from build123d import *

# Parameters (mm, degrees)
F0_R     = 2
F0_R_2   = 2.5
F2_DEPTH = 25


# Not quite as in the source:
# - ends of sketch curves that miss each other by under 0.0002 mm in the source are joined


with BuildPart() as f2:
    # F0 (on Front) → F2 (new body)
    with BuildSketch(Plane.XZ):
        with BuildLine():
            ThreePointArc((5.2500001607, 6.6439288361), (0, 4.5), (-5.2500001607, 6.6439288361))
            Line((-5.2500001607, 6.6439288361), (-5.25, 10.5))
            Line((-5.25, 10.5), (-3.375, 10.5))
            Line((-3.375, 10.5), (-3.375, 12.5))
            Line((-3.375, 12.5), (-7.5, 12.5))
            ThreePointArc((-7.5, 12.5), (-11.0355339059, 11.0355339059), (-12.5, 7.5))
            Line((-12.5, 7.5), (-12.5, 3.375))
            Line((-12.5, 3.375), (-10.5, 3.375))
            Line((-10.5, 3.375), (-10.5, 5.25))
            Line((-10.5, 5.25), (-6.643929, 5.25))
            ThreePointArc((-6.643929, 5.25), (-4.5, 0), (-6.6439288361, -5.2500001607))
            Line((-6.6439288361, -5.2500001607), (-10.5, -5.25))
            Line((-10.5, -5.25), (-10.5, -3.375))
            Line((-10.5, -3.375), (-12.5, -3.375))
            Line((-12.5, -3.375), (-12.5, -7.5))
            ThreePointArc((-12.5, -7.5), (-11.0355339059, -11.0355339059), (-7.5, -12.5))
            Line((-7.5, -12.5), (-3.375, -12.5))
            Line((-3.375, -12.5), (-3.375, -10.5))
            Line((-3.375, -10.5), (-5.25, -10.5))
            Line((-5.25, -10.5), (-5.25, -6.643929))
            ThreePointArc((-5.25, -6.643929), (0, -4.5), (5.2500001607, -6.6439288361))
            Line((5.2500001607, -6.6439288361), (5.25, -10.5))
            Line((5.25, -10.5), (3.375, -10.5))
            Line((3.375, -10.5), (3.375, -12.5))
            Line((3.375, -12.5), (7.5, -12.5))
            ThreePointArc((7.5, -12.5), (11.0355339059, -11.0355339059), (12.5, -7.5))
            Line((12.5, -7.5), (12.5, -3.375))
            Line((12.5, -3.375), (10.5, -3.375))
            Line((10.5, -3.375), (10.5, -5.25))
            Line((10.5, -5.25), (6.643929, -5.25))
            ThreePointArc((6.643929, -5.25), (4.5, 0), (6.6439288361, 5.2500001607))
            Line((6.6439288361, 5.2500001607), (10.5, 5.25))
            Line((10.5, 5.25), (10.5, 3.375))
            Line((10.5, 3.375), (12.5, 3.375))
            Line((12.5, 3.375), (12.5, 7.5))
            ThreePointArc((12.5, 7.5), (11.0355339059, 11.0355339059), (7.5, 12.5))
            Line((7.5, 12.5), (3.375, 12.5))
            Line((3.375, 12.5), (3.375, 10.5))
            Line((3.375, 10.5), (5.25, 10.5))
            Line((5.25, 10.5), (5.2500001607, 6.6439288361))
        make_face()
        with Locations((-8.5, -8.5)):
            Circle(F0_R, mode=Mode.SUBTRACT)
        with Locations((8.5, -8.5)):
            Circle(F0_R, mode=Mode.SUBTRACT)
        with Locations((-8.5, 8.5)):
            Circle(F0_R, mode=Mode.SUBTRACT)
        Circle(F0_R_2, mode=Mode.SUBTRACT)
        with Locations((8.5, 8.5)):
            Circle(F0_R, mode=Mode.SUBTRACT)
    extrude(amount=F2_DEPTH)


solid = f2.part
Work out the finished part from the listing and answer in its coordinate system (mm). A direction names the side the tool comes from. Round coordinates to 2 decimals unless told otherwise and drop trailing zeros. Write each loop counter-clockwise with the first axis right and the second up, starting at its lowest first coordinate (ties: lowest second). Pieces come first, ordered by that corner, then holes.
1) A cutting plane is placed at A-A (x = 0). Give the vertices of the cut face in (y, z).
2) Given pin 1 Ø1 at (y, z) = (-14.5, 11.5) entering from +X; pin 2 Ø1.2 at (x, y) = (9, -8) entering from -Z; pin 3 Ø1.6 at (y, z) = (-8.5, -12) entering from -X, each flat-ended and moving along its own axis, determine where each tip first touches the part or whether it passes through.
3) A cutting plane is placed at D-D (z = 0). Give the vertices of the cut face in (x, y).
4) A cutting plane is placed at B-B (z = -8.5). Give the vertices of the cut face in (x, y).
5) The mould has two halves that part along X. Classify faces 5 (the cylindrical face through (11, -12.32, -11.07)), 6 (the flat face through (5.25, -12, -9)), 7 (the flat face through (-5, -12, -12.5)): pulls with the +X half, pulls with the -X half, needs draft (parallel to the pull), parting line crosses it, or undercut.
6) A tool of negligible diameter and unlimited length cuts with its end or side. For faces 1 (the flat face through (11, -12, 3.375)), 2 (the flat face through (-3.375, -12, -12)), 3 (the flat face through (-5.25, -12, 9)), 4 (the flat face through (3.375, -12, 12)), from which of +Z, -Z, +X, -X, +Y, -Y can it reach the whole face along a straight path? Write none if from no direction.
7) A cutting plane is placed at C-C (x = 9). Give the vertices of the cut face in (y, z).
8) Straight lines are drawn through the part: line 1 (Z direction, x = 8.5, y = -16); line 2 (Z direction, x = -11.5, y = -4) (3 decimals); line 3 (Z direction, x = -8, y = -13). For each, find the intervals that lie inside material, in ascending order.
Completed:
1. outline: (-25, -4.5) - (0, -4.5) - (0, -2.5) - (-25, -2.5) - close; (-25, 2.5) - (0, 2.5) - (0, 4.5) - (-25, 4.5) - close
2. pin 1: stops at x = 11.07
2. pin 2: stops at z = -12.42
2. pin 3: stops at x = -10.86
3. outline: (-4.5, -25) - (-2.5, -25) - (-2.5, 0) - (-4.5, 0) - close; (2.5, -25) - (4.5, -25) - (4.5, 0) - (2.5, 0) - close
4. outline: (-12.4, -25) - (-10.5, -25) - (-10.5, 0) - (-12.4, 0) - close; (-6.5, -25) - (-5.25, -25) - (-5.25, 0) - (-6.5, 0) - close; (5.25, -25) - (6.5, -25) - (6.5, 0) - (5.25, 0) - close; (10.5, -25) - (12.4, -25) - (12.4, 0) - (10.5, 0) - close
5. face 5: pulls with the +X half
5. face 6: undercut
5. face 7: needs draft
6. face 1: +X, +Y, -Y
6. face 2: -Z, +Y, -Y
6. face 3: +Y, -Y
6. face 4: +Z, +Y, -Y
7. outline: (-25, -12.27) - (0, -12.27) - (0, -10.44) - (-25, -10.44) - close; (-25, -6.56) - (0, -6.56) - (0, -5.25) - (-25, -5.25) - close; (-25, 5.25) - (0, 5.25) - (0, 6.56) - (-25, 6.56) - close; (-25, 10.44) - (0, 10.44) - (0, 12.27) - (-25, 12.27) - close
8. line 1: z = -12.4 to -10.5, -6.5 to -5.25, 5.25 to 6.5, 10.5 to 12.4
8. line 2: z = -10.5 to -3.375, 3.375 to 10.5
8. line 3: z = -12.47 to -10.44, -6.56 to -5.25, 5.25 to 6.56, 10.44 to 12.47
